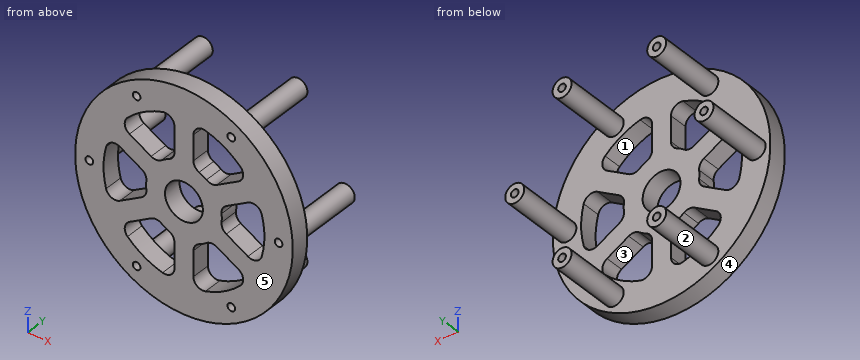
```python
from build123d import *

# Parameters (mm, degrees)
SKETCH1_R                  = 20
SKETCH1_R_2                = 10
BOSS_EXTRUDE1_DEPTH        = 5
SKETCH1_R_3                = 57.5
SKETCH1_R_4                = 42.5
BOSS_EXTRUDE1_2_DEPTH      = 5
SKETCH2_W                  = 10
SKETCH2_H                  = 32.5
BOSS_EXTRUDE2_DEPTH        = 10
SKETCH4_R                  = 5
BOSS_EXTRUDE3_DEPTH        = 36
TAP_DRILL_FOR_10_32_TAP1_D = 4.0386
FILLET1_R                  = 5
CIRPATTERN1_COUNT          = 6
FILLET1_OF_CIRPATTERN1_R   = 5


with BuildPart() as part:
    # Sketch1 → Boss-Extrude1 (new, symmetric)
    with BuildSketch(Plane(origin=(0, 0, 0), x_dir=(1, 0, 0), z_dir=(0, 1, 0))):
        with Locations(Location((0, 0, 0), (0, 0, 270))):
            Circle(SKETCH1_R)
        with Locations(Location((0, 0, 0), (0, 0, 270))):
            Circle(SKETCH1_R_2, mode=Mode.SUBTRACT)
    extrude(amount=BOSS_EXTRUDE1_DEPTH, both=True)



with BuildPart() as body_2:
    # Sketch1 → Boss-Extrude1 2 (new, symmetric)
    with BuildSketch(Plane(origin=(0, 0, 0), x_dir=(1, 0, 0), z_dir=(0, 1, 0))):
        with Locations(Location((0, 0, 0), (0, 0, 270))):
            Circle(SKETCH1_R_3)
        with Locations(Location((0, 0, 0), (0, 0, 270))):
            Circle(SKETCH1_R_4, mode=Mode.SUBTRACT)
    extrude(amount=BOSS_EXTRUDE1_2_DEPTH, both=True)


with BuildPart() as part_1:
    add(part.part)

    add(body_2.part)  # Boss-Extrude2 merges body 2
    # Sketch2 → Boss-Extrude2 (add)
    with BuildSketch(Plane.XZ.offset(5)):
        with Locations((0, 26.25)):
            Rectangle(SKETCH2_W, SKETCH2_H)
    boss_extrude2 = extrude(amount=-BOSS_EXTRUDE2_DEPTH)

    # Sketch4 → Boss-Extrude3 (add)
    with BuildSketch(Plane(origin=(0, 5, 0), x_dir=(1, 0, 0), z_dir=(0, 1, 0))):
        with Locations(Location((50, 0, 0), (0, 0, 270))):
            Circle(SKETCH4_R)
    boss_extrude3 = extrude(amount=BOSS_EXTRUDE3_DEPTH)

    # Tap Drill for #10-32 Tap1 (through all)
    with Locations(Plane(origin=(0, -5, 0), x_dir=(-1, 0, 0), z_dir=(0, -1, 0))):
        with Locations((-50, 0)):
            tap_drill_for_10_32_tap1 = Hole(TAP_DRILL_FOR_10_32_TAP1_D / 2)

    # Fillet1
    fillet1_edges = [part_1.edges().sort_by_distance(p)[0] for p in [
        (5, 0, 19.364916731),
        (-5, 0, 19.364916731),
        (5, 0, 42.20485754),
        (-5, 0, 42.20485754),
    ]]
    fillet(fillet1_edges, radius=FILLET1_R)

    # CirPattern1: Boss-Extrude2, Boss-Extrude3, Tap Drill for #10-32 Tap1 ×6 about axis
    cirpattern1_axis = Axis((0, 0, 0), (0, 1, 0))
    add([boss_extrude2.rotate(cirpattern1_axis, i * 360 / CIRPATTERN1_COUNT) for i in range(1, CIRPATTERN1_COUNT)])
    add([boss_extrude3.rotate(cirpattern1_axis, i * 360 / CIRPATTERN1_COUNT) for i in range(1, CIRPATTERN1_COUNT)])
    add([tap_drill_for_10_32_tap1.rotate(cirpattern1_axis, i * 360 / CIRPATTERN1_COUNT) for i in range(1, CIRPATTERN1_COUNT)], mode=Mode.SUBTRACT)

    # Fillet1 of CirPattern1
    fillet1_of_cirpattern1_edges = [part_1.edges().sort_by_distance(p)[0] for p in [
        (19.270509831, 0, 5.352331347),
        (14.270509831, 0, 14.012585384),
        (39.050478793, 0, 16.772301751),
        (34.050478793, 0, 25.432555789),
        (14.270509831, 0, -14.012585384),
        (19.270509831, 0, -5.352331347),
        (34.050478793, 0, -25.432555789),
        (39.050478793, 0, -16.772301751),
        (-5, 0, -19.364916731),
        (5, 0, -19.364916731),
        (-5, 0, -42.20485754),
        (5, 0, -42.20485754),
        (-19.270509831, 0, -5.352331347),
        (-14.270509831, 0, -14.012585384),
        (-39.050478793, 0, -16.772301751),
        (-34.050478793, 0, -25.432555789),
        (-14.270509831, 0, 14.012585384),
        (-19.270509831, 0, 5.352331347),
        (-34.050478793, 0, 25.432555789),
        (-39.050478793, 0, 16.772301751),
    ]]
    fillet(fillet1_of_cirpattern1_edges, radius=FILLET1_OF_CIRPATTERN1_R)


solid = part_1.part
```
Geometry check sheet. Reference: the model listing, model coordinates, mm. Face numbers are marked on the shaded views. A direction names the side the tool comes from. Coordinates: 2 decimals unless noted, no trailing zeros. Loops run counter-clockwise (first coordinate to the right, second up) from the corner with the lowest first, then second, coordinate; pieces in that order, holes last. Notation, with made-up numbers: (2, 24.5) - (11, 24.5) arc R17 cw to (11, 51.5) - close; hole circle Ø6 at (-32, 41). An arc over 180 degrees is marked (long way). One line per item, written item: value. Start each with the question number.
(1) Material ranges on line 1 (X direction, y = 18, z = -43); line 2 (Z direction, x = 14.5, y = 3); line 3 (Z direction, x = 19.5, y = -0.5), recorded low to high. Write a range as [from, to].
(2) Tool access check on the marked faces 1 and 2. Record the directions out of +Z, -Z, +X, -X, +Y, -Y that give a thin tool (end or side, any length) a straight path to the whole face; none if there is none.
(3) Depth check by flat-ended pin: P1, Ø8, axis at y = -0.5, z = 32, coming from the -X side; P2, Ø1, axis at x = 10.5, z = -43, coming from the +Y side; P3, Ø5, axis at y = 1.5, z = -30, coming from the +X side. Enter the tip coordinate at first touch or a pass-through.
(4) Cross-section at B-B on x = 0. Enter the section's corners in (y, z).
(5) Cross-section at A-A on y = 36.5. Count the separate pieces of the cut face and the enclosed holes in it, plus the area to 3 significant figures.
(6) Mould release check, pull along Z, two halves, no side actions. Record for the marked faces 3, 4 and 5: released by +Z, released by -Z, zero draft, split by the parting line, or undercut.
Results below:
1. line 1: x = [-29.99, -27], [-23, -20.01], [20.01, 23], [27, 29.99]
1. line 2: z = [-55.64, -39.95], [-15.13, 15.13], [39.95, 55.64]
1. line 3: z = [-54.09, -37.76], [-17.03, 17.03], [37.76, 54.09]
2. face 1: +Y, -Y
2. face 2: +Y
3. P1: stops at x = -50.22
3. P2: stops at y = 5
3. P3: stops at x = 50.5
4. outline: (-5, -57.5) - (5, -57.5) - (5, -10) - (-5, -10) - close; (-5, 10) - (5, 10) - (5, 57.5) - (-5, 57.5) - close
5. separate pieces: 6
5. enclosed holes: 6
5. area: 394 mm2
6. face 3: undercut
6. face 4: split by the parting line
6. face 5: zero draft
